The drawing under review shows one solid part. Ordinate dimensions are in mm from its lowest x, y, z. Coordinates: 2 decimals unless noted, no trailing zeros. Write each loop counter-clockwise with the first axis right and the second up, starting at its lowest first coordinate (ties: lowest second). Pieces come first, ordered by that corner, then holes.
1) For line 1 (X direction, y = 6.25, z = 9); line 2 (Y direction, x = 11, z = 19); line 3 (X direction, y = 11, z = 6.5), list the stretches that pass through material, from the lowest coordinate up.
2) Mouldability with a two-part tool opening along X and no side actions: class the marked faces 1, 2, 3 and 4 as released by +X, released by -X, zero draft, split by the parting line, or undercut.
3) For P1, Ø1.5, axis at x = 5.5, z = 7.5, coming from the -Y side (1 decimal); P2, Ø6.5, axis at x = 18.5, z = 21.5, coming from the +Y side; P3, Ø12, axis at x = 19, y = 23.5, coming from the +Z side, all flat-tipped, find the tip position at first contact; note any pin that passes through.
4) Add section D-D, the plane y = 22.25. State the section outline as (x, z) points, then the cut area to 3 significant figures.
5) Add section A-A, the plane y = 7. State the section outline as (x, z) points, then the cut area to 3 significant figures.
6) Add section B-B, the plane x = 28.5. State the section outline as (y, z) points (1 decimal).
7) Add section C-C, the plane z = 22. State the section outline as (x, y) points, then the cut area to 3 significant figures.
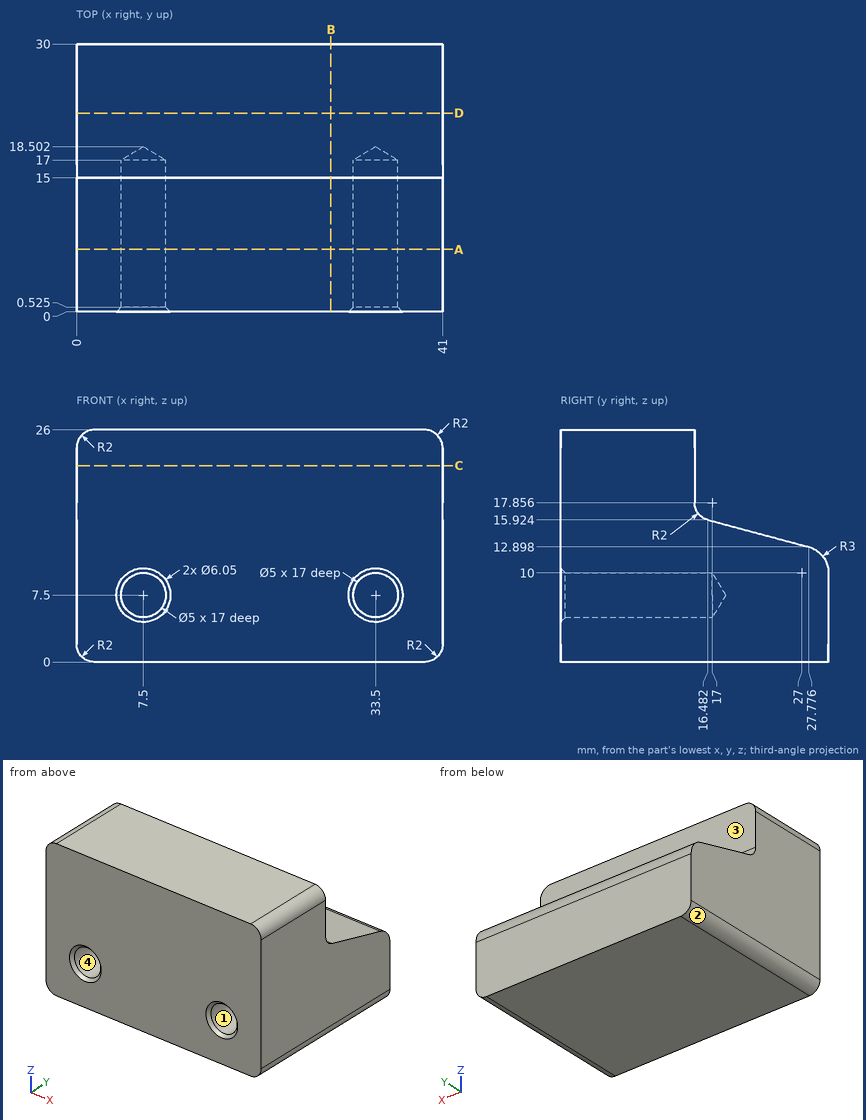
Geometry results:
1. line 1: x = 0 to 5.5, 9.5 to 31.5, 35.5 to 41
1. line 2: y = 0 to 15
1. line 3: x = 0 to 5.21, 9.79 to 31.21, 35.79 to 41
2. face 1: undercut
2. face 2: released by -X
2. face 3: zero draft
2. face 4: undercut
3. P1: stops at y = 0.3
3. P2: stops at y = 15
3. P3: stops at z = 15.65
4. outline: (0, 2) arc R2 ccw to (2, 0) - (39, 0) arc R2 ccw to (41, 2) - (41, 14.38) - (0, 14.38) - close
4. area: 588 mm2
5. outline: (0, 2) arc R2 ccw to (2, 0) - (39, 0) arc R2 ccw to (41, 2) - (41, 24) arc R2 ccw to (39, 26) - (2, 26) arc R2 ccw to (0, 24) - close; hole circle Ø5 at (7.5, 7.5); hole circle Ø5 at (33.5, 7.5)
5. area: 1,020 mm2
6. outline: (0, 0) - (30, 0) - (30, 10) arc R3 ccw to (27.8, 12.9) - (16.5, 15.9) arc R2 cw to (15, 17.9) - (15, 26) - (0, 26) - close
7. outline: (0, 0) - (41, 0) - (41, 15) - (0, 15) - close
7. area: 615 mm2
